The listing builds one solid part. Answer for the finished solid, in the listing's coordinates (mm). Face numbers are marked on the shaded views. A direction names the side the tool comes from. Round coordinates to 2 decimals unless told otherwise and drop trailing zeros. Loops run counter-clockwise (first coordinate to the right, second up) from the corner with the lowest first, then second, coordinate; pieces in that order, holes last. Notation, with made-up numbers: M 41.25,32.25 L 52.25,32.25 A29 ccw 52.25,62.25 Z; hole C 51.25,60.25 d6. An arc over 180 degrees is marked long. Put each result on its own line as item: value. Start each with the question number.
(1) Section C-C, the plane z = -3 is taken. Determine the outline of the cut face in (x, y), then the cut area to 3 significant figures.
(2) Section B-B, the plane y = -7 is taken. Count the separate pieces of the cut face and the enclosed holes in it, then the cut area to 3 significant figures.
(3) Straight lines are drawn through the part: line 1 (X direction, y = -5.25, z = -20); line 2 (X direction, y = -6.5, z = -24.5); line 3 (X direction, y = -7.5, z = -20.5). For each, find the intervals that lie inside material, in ascending order.
(4) Flat-ended cylindrical pins translate along their axes: P1, Ø1, axis at x = -3, y = -1, coming from the -Z side; P2, Ø4, axis at x = -12.5, y = -1, coming from the +Z side; P3, Ø1, axis at x = -12.5, y = -4, coming from the -Z side. Find the tip coordinate at first contact, or state that the pin passes through.
(5) Section D-D, the plane x = 8 is taken. Determine the outline of the cut face in (y, z).
(6) Determine the mould class of the marked faces 4, 5 and 6 for opening direction Z: released by +Z, released by -Z, zero draft, split by the parting line, or undercut.
(7) Section A-A, the plane x = 1 is taken. Determine the outline of the cut face in (y, z), then the cut area to 3 significant figures.
(8) Which of the six approach directions +Z, -Z, +X, -X, +Y, -Y give full straight-line access (tool end or side, diameter ignored) to the marked faces 1, 2 and 3?
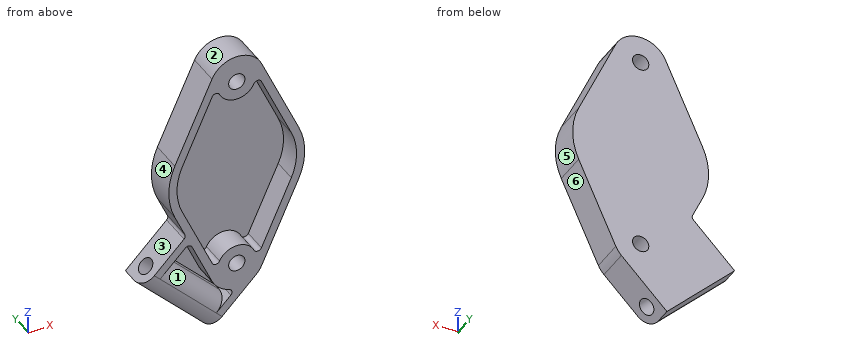
```python
from build123d import *

# Parameters (mm, degrees)
F0_R     = 2
F1_DEPTH = 8
F2_DEPTH = 2
F3_R     = 1
F5_D     = 4
F6_R     = 3.99999


# Not quite as in the source:
# - a fillet or chamfer is up to 0.001 mm smaller than in the source, because OpenCascade refuses the exact size


with BuildPart() as f1:
    # F0 (on Front) → F1 (new body)
    with BuildSketch(Plane.XZ):
        with BuildLine():
            Line((15.1970139668, 6.8636525628), (6.0880650012, 27.0320429916))
            ThreePointArc((6.0880650012, 27.0320429916), (0, 30.9626), (-6.0880650012, 27.0320429916))
            Line((-6.0880650012, 27.0320429916), (-15.1970139668, 6.8636525628))
            ThreePointArc((-15.1970139668, 6.8636525628), (-16.6751, 0), (-15.1970139668, -6.8636525628))
            Line((-15.1970139668, -6.8636525628), (-12.4500889322, -12.9456996558))
            Line((-12.4500889322, -12.9456996558), (-11.570090993, -14.8941288413))
            Line((-11.570090993, -14.8941288413), (-6.0880650012, -27.0320429916))
            ThreePointArc((-6.0880650012, -27.0320429916), (-3.6489564687, -29.8779507977), (-0.0611180905, -30.9623204051))
            ThreePointArc((-0.0611180905, -30.9623204051), (2.5281419438, -30.4657300374), (4.7236147197, -29.0060147197))
            ThreePointArc((4.7236147197, -29.0060147197), (5.4952020611, -28.0807978659), (6.0880650012, -27.0320429916))
            Line((6.0880650012, -27.0320429916), (15.1970139668, -6.8636525628))
            ThreePointArc((15.1970139668, -6.8636525628), (16.6751, 0), (15.1970139668, 6.8636525628))
        make_face()
        with Locations((0, -24.2824)):
            Circle(F0_R, mode=Mode.SUBTRACT)
        with BuildLine():
            Line((-13.3742945868, 6.0404308054), (-6.0462846285, 22.2655920687))
            ThreePointArc((-6.0462846285, 22.2655920687), (-5.1436901116, 22.8539427752), (-4.2309206889, 22.2815046593))
            ThreePointArc((-4.2309206889, 22.2815046593), (0, 19.6022), (4.2309206889, 22.2815046593))
            ThreePointArc((4.2309206889, 22.2815046593), (5.1436901116, 22.8539427752), (6.0462846285, 22.2655920687))
            Line((6.0462846285, 22.2655920687), (13.3742945868, 6.0404308054))
            ThreePointArc((13.3742945868, 6.0404308054), (14.6751, 0), (13.3742945868, -6.0404308054))
            Line((13.3742945868, -6.0404308054), (6.0462846285, -22.2655920687))
            ThreePointArc((6.0462846285, -22.2655920687), (5.1436901116, -22.8539427752), (4.2309206889, -22.2815046593))
            ThreePointArc((4.2309206889, -22.2815046593), (0, -19.6022), (-4.2309206889, -22.2815046593))
            ThreePointArc((-4.2309206889, -22.2815046593), (-5.1436901116, -22.8539427752), (-6.0462846285, -22.2655920687))
            Line((-6.0462846285, -22.2655920687), (-13.3742945868, -6.0404308054))
            ThreePointArc((-13.3742945868, -6.0404308054), (-14.6751, 0), (-13.3742945868, 6.0404308054))
        make_face(mode=Mode.SUBTRACT)
        with Locations((0, 24.2824)):
            Circle(F0_R, mode=Mode.SUBTRACT)
        with BuildLine():
            Line((-11.570090993, -14.8941288413), (-12.4500889322, -12.9456996558))
            Line((-12.4500889322, -12.9456996558), (-23.05669065, -23.5523013736))
            Line((-23.05669065, -23.5523013736), (-6.4396812921, -40.1693107315))
            Line((-6.4396812921, -40.1693107315), (4.7236147197, -29.0060147197))
            ThreePointArc((4.7236147197, -29.0060147197), (2.5281419438, -30.4657300374), (-0.0611180905, -30.9623204051))
            Line((-0.0611180905, -30.9623204051), (-2.197040605, -33.0982429196))
            Line((-2.197040605, -33.0982429196), (-15.9856228381, -19.3096606865))
            Line((-15.9856228381, -19.3096606865), (-11.570090993, -14.8941288413))
        make_face()
    extrude(amount=F1_DEPTH)

    # F0 (on Front) → F2 (join)
    with BuildSketch(Plane.XZ):
        with BuildLine():
            ThreePointArc((-4.2309206889, 22.2815046593), (-5.1436901116, 22.8539427752), (-6.0462846285, 22.2655920687))
            Line((-6.0462846285, 22.2655920687), (-13.3742945868, 6.0404308054))
            ThreePointArc((-13.3742945868, 6.0404308054), (-14.6751, 0), (-13.3742945868, -6.0404308054))
            Line((-13.3742945868, -6.0404308054), (-6.0462846285, -22.2655920687))
            ThreePointArc((-6.0462846285, -22.2655920687), (-5.1436901116, -22.8539427752), (-4.2309206889, -22.2815046593))
            ThreePointArc((-4.2309206889, -22.2815046593), (0, -19.6022), (4.2309206889, -22.2815046593))
            ThreePointArc((4.2309206889, -22.2815046593), (5.1436901116, -22.8539427752), (6.0462846285, -22.2655920687))
            Line((6.0462846285, -22.2655920687), (13.3742945868, -6.0404308054))
            ThreePointArc((13.3742945868, -6.0404308054), (14.6751, 0), (13.3742945868, 6.0404308054))
            Line((13.3742945868, 6.0404308054), (6.0462846285, 22.2655920687))
            ThreePointArc((6.0462846285, 22.2655920687), (5.1436901116, 22.8539427752), (4.2309206889, 22.2815046593))
            ThreePointArc((4.2309206889, 22.2815046593), (0, 19.6022), (-4.2309206889, 22.2815046593))
        make_face()
        with BuildLine():
            Line((-6.0880650012, -27.0320429916), (-11.570090993, -14.8941288413))
            Line((-11.570090993, -14.8941288413), (-15.9856228381, -19.3096606865))
            Line((-15.9856228381, -19.3096606865), (-2.197040605, -33.0982429196))
            Line((-2.197040605, -33.0982429196), (-0.0611180905, -30.9623204051))
            ThreePointArc((-0.0611180905, -30.9623204051), (-3.6489564687, -29.8779507977), (-6.0880650012, -27.0320429916))
        make_face()
    extrude(amount=F2_DEPTH)

    # F3
    f3_edges = [f1.edges().sort_by_distance(p)[0] for p in [
        (-12.450089, -4, -12.9457),
        (-11.570091, -5, -14.894129),
        (-0.061118, -5, -30.96232),
    ]]
    fillet(f3_edges, radius=F3_R)

    # F5 (through all)
    with Locations(Plane(origin=(16.8648147197, 0, -16.8648147197), x_dir=(0, 1, 0), z_dir=(0.7071067812, 0, -0.7071067812))):
        with Locations((-4, -28.9575343242)):
            Hole(F5_D / 2)

    # F6 (radius 4 in the source; OpenCascade refuses exactly that, so slightly less here)
    f6_edges = [f1.edges().sort_by_distance(p)[0] for p in [
        (-14.748186, -8, -31.860806),
        (-9.091332, -8, -26.203952),
    ]]
    fillet(f6_edges, radius=F6_R)


solid = f1.part
```
Recorded:
1. outline: M -16.4,-8 L -14.37,-8 L -14.37,-2 L 14.37,-2 L 14.37,-8 L 16.4,-8 L 16.4,0 L -16.4,0 Z
1. area: 90.1 mm²
2. separate pieces: 1
2. enclosed holes: 4
2. area: 555 mm²
3. line 1: x = -18.74 to -15.58, -9.26 to -7.07, -1.89 to 1.89, 7.07 to 9.26
3. line 2: x = -20.87 to -12.04, -7.23 to -1.99, 1.99 to 7.23
3. line 3: x = -20 to -17.18, -9.04 to -6.84, -2.76 to 2.76, 6.84 to 9.04
4. P1: stops at z = -37.23
4. P2: stops at z = 17.26
4. P3: stops at z = -34.61
5. outline: M -8,-22.8 L 0,-22.8 L 0,22.8 L -8,22.8 L -8,17.94 L -2,17.94 L -2,-17.94 L -8,-17.94 Z
6. face 4: undercut
6. face 5: split by the parting line
6. face 6: released by -Z
7. outline: M -8,-32.73 L 0,-32.73 L 0,-26.01 L -8,-26.01 Z; M -8,-22.55 L 0,-22.55 L 0,22.55 L -8,22.55 L -8,19.71 L -2,19.71 L -2,-19.71 L -8,-19.71 Z; M -8,26.01 L 0,26.01 L 0,30.89 L -8,30.89 Z
7. area: 217 mm²
8. face 1: -Y
8. face 2: +Z, +Y, -Y
8. face 3: -X, +Y, -Y
